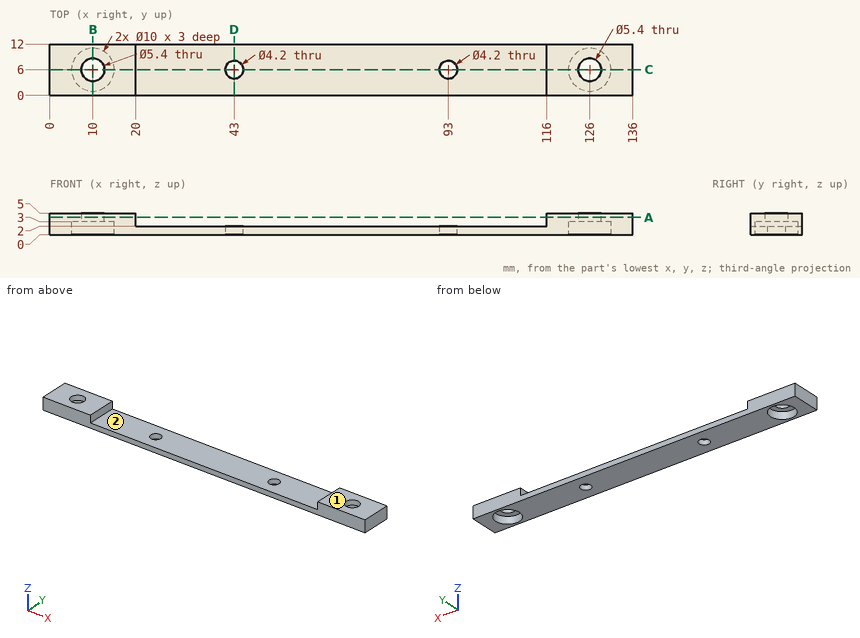
Geometry: see drawing. Coordinates: mm, zero at the bounding-box minimum. Give positions to 0.01 mm unless a question says otherwise; leave off trailing zeros. Order: outer loops, then holes, each group sorted by start corner. A loop starts at its lowest first (then second) coordinate and runs counter-clockwise, first axis right, second up.
Q1. Contact query for flat-ended pins moving along their axis: pin 1 Ø3.5 at (x, y) = (60, 8.5) entering from +Z; pin 2 Ø3 at (x, y) = (11, 8) entering from -Z. Output: stop coordinate, or through.
Checked values:
pin 1: stops at z = 2
pin 2: stops at z = 3
Q2. Draft query along X for the marked faces 1 and 2. Return one class per face: +X half, -X half, draft (parallel to the pull), parting line (faces both ways), or undercut.
Checked values:
face 1: draft
face 2: undercut
Q3. Section B-B on x = 10. Output: boundary loops of the cut face in (y, z).
Checked values:
outline: (0, 0) - (1, 0) - (1, 3) - (3.3, 3) - (3.3, 5) - (0, 5) - close; (8.7, 3) - (11, 3) - (11, 0) - (12, 0) - (12, 5) - (8.7, 5) - close
Q4. Ray query, probe 1 along X at (y, z) = (6, 3.5); probe 2 along X at (y, z) = (10.25, 1.1); probe 3 along X at (y, z) = (9, 1.4). Return the intervals inside material, ascending.
Checked values:
probe 1: x = 0 to 7.3, 12.7 to 20, 116 to 123.3, 128.7 to 136
probe 2: x = 0 to 7.37, 12.63 to 123.37, 128.63 to 136
probe 3: x = 0 to 6, 14 to 122, 130 to 136
Q5. Section A-A on z = 4.1. Output: boundary loops of the cut face in (x, y), and give its area (3 significant figures).
Checked values:
outline: (0, 0) - (20, 0) - (20, 12) - (0, 12) - close; (116, 0) - (136, 0) - (136, 12) - (116, 12) - close; hole circle Ø5.4 at (10, 6); hole circle Ø5.4 at (126, 6)
area: 434 mm2
Q6. Section C-C on y = 6. State how many separate pieces and enclosed holes the cut face has, and give its area (3 significant figures).
Checked values:
separate pieces: 5
enclosed holes: 0
area: 294 mm2
Q7. Section D-D on x = 43. Output: boundary loops of the cut face in (y, z).
Checked values:
outline: (0, 0) - (3.9, 0) - (3.9, 2) - (0, 2) - close; (8.1, 0) - (12, 0) - (12, 2) - (8.1, 2) - close
